Could you check a few things on this model? Use its own coordinates, in mm. Face numbers are marked on the shaded views. A direction names the side the tool comes from. Give positions to 0.01 mm unless a question says otherwise; leave off trailing zeros. One line per item, written item: value.
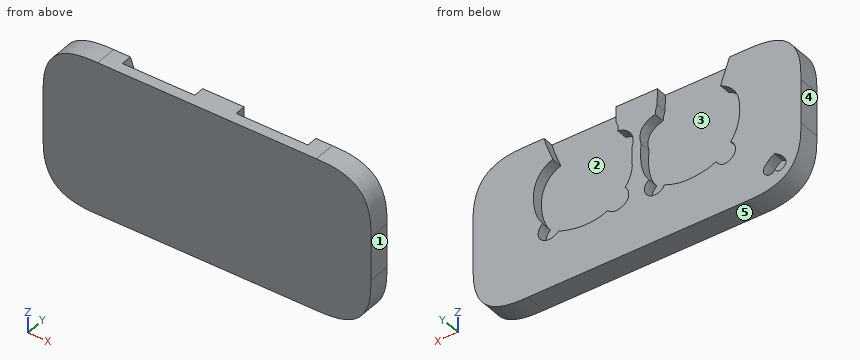
```python
from build123d import *

# Parameters (mm, degrees)
SKETCH_1_W          = 60
SKETCH_1_H          = 28
EXTRUDE_1_DEPTH     = 4
FILLET_1_SIZE       = 10
CUT_EXTRUDE_1_DEPTH = 2


with BuildPart() as part:
    # 草图1 → 凸台-拉伸1 (new body)
    with BuildSketch(Plane(origin=(0, 0, 0), x_dir=(1, 0, 0), z_dir=(0, 1, 0))):
        Rectangle(SKETCH_1_W, SKETCH_1_H)
    extrude(amount=EXTRUDE_1_DEPTH)

    # 圆角1
    # a fillet whose section is not a circle: 10 mm, written as the material it takes off along each edge
    with BuildSketch(Plane(origin=(30, -25, 14), x_dir=(0, 0, -1), z_dir=(0, 1, 0)), Plane(origin=(30, -25, -14), x_dir=(-1, 0, 0), z_dir=(0, 1, 0)), Plane(origin=(-30, -25, 14), x_dir=(1, 0, 0), z_dir=(0, 1, 0))) as fillet_1_piece_1:
        with BuildLine():
            add(Edge.make_bspline([(FILLET_1_SIZE, 0), (FILLET_1_SIZE * 0.831801948466, 0), (FILLET_1_SIZE * 0.663603896932, 0), (FILLET_1_SIZE * 0.292893218813, FILLET_1_SIZE * 0.0716919198361), (FILLET_1_SIZE * 0.0716919198361, FILLET_1_SIZE * 0.292893218813), (0, FILLET_1_SIZE * 0.663603896932), (0, FILLET_1_SIZE * 0.831801948466), (0, FILLET_1_SIZE)], knots=[0, 0, 0, 0, 0, 0, 0.5, 0.5, 1, 1, 1, 1, 1, 1], degree=5))
            Line((0, FILLET_1_SIZE), (0, 0))
            Line((0, 0), (FILLET_1_SIZE, 0))
        make_face()
    extrude(amount=54, mode=Mode.SUBTRACT)
    with BuildSketch(Plane(origin=(-30, -25, -14), x_dir=(1, 0, 0), z_dir=(0, 1, 0))) as fillet_1_piece_2:
        with BuildLine():
            add(Edge.make_bspline([(FILLET_1_SIZE, 0), (FILLET_1_SIZE * 0.831801948466, 0), (FILLET_1_SIZE * 0.663603896932, 0), (FILLET_1_SIZE * 0.292893218813, -FILLET_1_SIZE * 0.0716919198361), (FILLET_1_SIZE * 0.0716919198361, -FILLET_1_SIZE * 0.292893218813), (0, -FILLET_1_SIZE * 0.663603896932), (0, -FILLET_1_SIZE * 0.831801948466), (0, -FILLET_1_SIZE)], knots=[0, 0, 0, 0, 0, 0, 0.5, 0.5, 1, 1, 1, 1, 1, 1], degree=5))
            Line((0, -FILLET_1_SIZE), (0, 0))
            Line((0, 0), (FILLET_1_SIZE, 0))
        make_face()
    extrude(amount=54, mode=Mode.SUBTRACT)

    # 草图2 → 切除-拉伸1 (cut)
    with BuildSketch(Plane(origin=(0, 4, 0), x_dir=(1, 0, 0), z_dir=(0, 1, 0))):
        with BuildLine():
            Line((-16.935076069, -14), (-3.724944257, -14))
            add(Edge.make_bspline(
                [(-3.687819463, -11.10018183), (-3.670837845, -12.550695913), (-3.724944257, -14)],
                knots=[0, 0, 0, 1, 1, 1], degree=2))
            add(Edge.make_bspline(
                [(-3.333312713, -9.429337618), (-3.330795543, -10.302670918), (-3.687819463, -11.10018183)],
                knots=[0, 0, 0, 1, 1, 1], degree=2))
            add(Edge.make_bspline(
                [(-0.742711054, -5.127809832), (-0.519156675, -5.880287043), (-0.292936969, -8.050568721), (-2.341442668, -9.22030854), (-3.333312713, -9.429337618)],
                knots=[0, 0, 0, 0, 0.428917256, 1, 1, 1, 1], degree=3))
            add(Edge.make_bspline(
                [(-2.187125143, 2.12230749), (-1.4106002, 1.204552618), (-0.592489001, -1.244047904), (-0.600668316, -3.791601167), (-0.742711054, -5.127809832)],
                knots=[0, 0, 0, 0, 0.466812094, 1, 1, 1, 1], degree=3))
            add(Edge.make_bspline(
                [(-4.963765819, 4.30996378), (-4.793040938, 4.977205844), (-3.75279166, 5.532669201), (-2.278151789, 5.341305653), (-1.531570873, 4.465738286), (-1.148751049, 3.242289174), (-1.743465674, 2.389914822), (-2.187125143, 2.12230749)],
                knots=[0, 0, 0, 0, 0.278653368, 0.467417998, 0.60771691, 0.765483941, 1, 1, 1, 1], degree=3))
            add(Edge.make_bspline(
                [(-14.443609745, 4.225823154), (-13.661769199, 4.701986871), (-12.07963713, 5.088608477), (-9.80873584, 5.325514917), (-7.438485821, 5.235768859), (-5.859496423, 4.683683956), (-4.963765819, 4.30996378)],
                knots=[0, 0, 0, 0, 0.277671681, 0.493980308, 0.700924653, 1, 1, 1, 1], degree=3))
            add(Edge.make_bspline(
                [(-17.112369797, 1.740167248), (-17.796876509, 2.159176308), (-18.361225861, 3.59646204), (-17.356865882, 4.881210301), (-16.40295998, 5.370009473), (-15.208277597, 5.256104096), (-14.685195355, 4.587656422), (-14.443609745, 4.225823154)],
                knots=[0, 0, 0, 0, 0.353240726, 0.517926677, 0.663976899, 0.804852125, 1, 1, 1, 1], degree=3))
            add(Edge.make_bspline(
                [(-15.280334608, -9.429337618), (-16.497678509, -8.866325433), (-18.294247529, -7.346930593), (-18.872884283, -4.315150537), (-18.745655148, -1.369033801), (-17.944096186, 0.728594057), (-17.112369797, 1.740167248)],
                knots=[0, 0, 0, 0, 0.318174296, 0.494604613, 0.698392994, 1, 1, 1, 1], degree=3))
            Line((-15.280334608, -9.429337618), (-16.935076069, -14))
        make_face()
        with BuildLine():
            Line((3.859545005, -14), (16.989453484, -14))
            add(Edge.make_bspline(
                [(15.404911602, -9.429337618), (15.900430103, -10.960211179), (16.69378742, -12.407476359), (16.989453484, -14)],
                knots=[0, 0, 0, 0, 1, 1, 1, 1], degree=3))
            add(Edge.make_bspline(
                [(17.288668554, 1.574170629), (18.287334611, 0.305452853), (19.081858131, -2.363427448), (18.899603104, -6.766539361), (16.920972519, -8.986056385), (15.404911602, -9.429337618)],
                knots=[0, 0, 0, 0, 0.370985391, 0.64043209, 1, 1, 1, 1], degree=3))
            add(Edge.make_bspline(
                [(14.333173858, 4.30996378), (14.813620622, 4.805305608), (15.919659705, 5.273598818), (17.423209254, 4.783697576), (18.393133704, 3.377287394), (17.886541605, 2.047965808), (17.288668554, 1.574170629)],
                knots=[0, 0, 0, 0, 0.305299637, 0.480890731, 0.659706763, 1, 1, 1, 1], degree=3))
            add(Edge.make_bspline(
                [(5.359934346, 4.464221596), (8.147654076, 5.822153518), (11.537691595, 5.354629666), (14.333173858, 4.30996378)],
                knots=[0, 0, 0, 0, 1, 1, 1, 1], degree=3))
            add(Edge.make_bspline(
                [(2.170811741, 1.574170629), (1.581087403, 2.132858214), (1.138470768, 3.878747123), (3.169357766, 5.317866652), (4.664971625, 5.28325304), (5.359934346, 4.464221596)],
                knots=[0, 0, 0, 0, 0.379311018, 0.599175154, 1, 1, 1, 1], degree=3))
            add(Edge.make_bspline(
                [(0.941523625, -5.262232932), (0.98567745, -3.887367548), (0.523188823, -1.466699515), (1.521155106, 0.830396312), (2.170811741, 1.574170629)],
                knots=[0, 0, 0, 0, 0.583806076, 1, 1, 1, 1], degree=3))
            add(Edge.make_bspline(
                [(3.524384204, -9.429337618), (2.557976333, -9.282877204), (1.192253003, -8.451499296), (0.573882177, -6.601892019), (0.759159881, -5.696024028), (0.941523625, -5.262232932)],
                knots=[0, 0, 0, 0, 0.526961764, 0.748177959, 1, 1, 1, 1], degree=3))
            add(Edge.make_bspline(
                [(3.821968614, -11.10018183), (3.337919448, -10.344678931), (3.524384204, -9.429337618)],
                knots=[0, 0, 0, 1, 1, 1], degree=2))
            add(Edge.make_bspline(
                [(3.859545005, -14), (3.769556535, -12.550344491), (3.821968614, -11.10018183)],
                knots=[0, 0, 0, 1, 1, 1], degree=2))
        make_face()
        with BuildLine():
            add(Edge.make_bspline(
                [(-25.185013425, 10.431735443), (-25.689297318, 11.557258243), (-28.770586094, 10.040399625), (-25.818873431, 7.748418433), (-25.185013425, 7.531774201)],
                knots=[0, 0, 0, 0, 0.419335828, 1, 1, 1, 1], degree=3))
            add(Edge.make_bspline(
                [(-25.185013425, 10.431735443), (-24.680729531, 11.557258243), (-21.599440755, 10.040399625), (-24.551153418, 7.748418433), (-25.185013425, 7.531774201)],
                knots=[0, 0, 0, 0, 0.419335828, 1, 1, 1, 1], degree=3))
        make_face()
    extrude(amount=-CUT_EXTRUDE_1_DEPTH, mode=Mode.SUBTRACT)


solid = part.part
```
1) Please list where these lines run through material, in increasing order: L1, parallel to X at y = 2.75, z = 0.5; L2, parallel to X at y = 2.25, z = 2; L3, parallel to Y at x = -4.5, z = 12.5. Write a range as from..to.
Outcome:
L1: x = -30..-18.32, -0.95..1.08, 18.41..30
L2: x = -30..-18.68, -0.71..0.86, 18.79..30
L3: y = 0..2
2) I'm going to push flat-ended pins straight in: pin 1 (1.5 mm diameter, centred on y = 2.5, z = -8.5, fed in from -X); pin 2 (1 mm diameter, centred on y = 0.5, z = 9.5, fed in from +X); pin 3 (9 mm diameter, centred on x = 8.5, z = 0, fed in from +Y). Where does each tip first touch, or does it pass through?
Outcome:
pin 1: stops at x = -29.75
pin 2: stops at x = 29.44
pin 3: stops at y = 2
3) We'd pull the mould along Z, two halves only. Please class the marked faces 3, 4 and 5: pulls with the +Z half, pulls with the -Z half, needs draft (parallel to the pull), parting line crosses it, or undercut.
Outcome:
face 3: undercut
face 4: needs draft
face 5: pulls with the -Z half
4) On a 3-axis mill with a long thin cutter (end or side, diameter ignored), from which of +Z, -Z, +X, -X, +Y, -Y can I reach the whole of each face in a straight line? I mean the marked faces 1 and 2. Say none if no direction works.
Outcome:
face 1: +Z, -Z, +X, +Y, -Y
face 2: +Y
